from build123d import *

# Parameters (mm, degrees)
EXTRUDE_1_DEPTH     = 6.8
CUT_EXTRUDE_1_DEPTH = 6.9
SKETCH_3_W          = 104
SKETCH_3_H          = 28
EXTRUDE_2_DEPTH     = 32.2
SKETCH_4_W          = 27.8
SKETCH_4_H          = 4.8
CUT_EXTRUDE_2_DEPTH = 6
SKETCH_4_3_W        = 27.8
SKETCH_4_3_H        = 4.8
EXTRUDE_3_DEPTH     = 6
SKETCH_5_W          = 14
SKETCH_5_H          = 14
CUT_EXTRUDE_3_DEPTH = 14
SKETCH_6_R          = 4.2
CUT_EXTRUDE_4_DEPTH = 155.304892988
FILLET_1_R          = 14


with BuildPart() as part:
    # Эскиз1 → Бобышка-Вытянуть1 (new body)
    with BuildSketch(Plane(origin=(0, 0, 0), x_dir=(1, 0, 0), z_dir=(0, 1, 0))):
        with BuildLine():
            ThreePointArc((-28, 0), (0, -28), (28, 0))
            ThreePointArc((28, 0), (11.895099372, 40.186413418), (-28, 57))
            Line((-28, 57), (-140, 57))
            Line((-140, 57), (-140, 29))
            Line((-140, 29), (-36, 29))
            ThreePointArc((-36, 29), (-30.343145751, 26.656854249), (-28, 21))
            Line((-28, 21), (-28, 0))
        make_face()
    extrude(amount=EXTRUDE_1_DEPTH)

    # Эскиз2 → Вырез-Вытянуть1 (cut)
    with BuildSketch(Plane(origin=(0, 6.8, 0), x_dir=(1, 0, 0), z_dir=(0, 1, 0))):
        Polygon((0, 7.15), (-6.192081637, 3.575), (-6.192081637, -3.575), (0, -7.15), (6.192081637, -3.575), (6.192081637, 3.575), align=None)
    extrude(amount=-CUT_EXTRUDE_1_DEPTH, mode=Mode.SUBTRACT)

    # Эскиз3 → Бобышка-Вытянуть2 (add)
    with BuildSketch(Plane(origin=(0, 6.8, 0), x_dir=(1, 0, 0), z_dir=(0, 1, 0))):
        with Locations((-88, 43)):
            Rectangle(SKETCH_3_W, SKETCH_3_H)
    extrude(amount=EXTRUDE_2_DEPTH)

    # Эскиз4 → Вырез-Вытянуть2 (cut)
    with BuildSketch(Plane(origin=(0, 39, 0), x_dir=(1, 0, 0), z_dir=(0, 1, 0))):
        with Locations((-56, 48.6)):
            Rectangle(SKETCH_4_W, SKETCH_4_H)
    extrude(amount=-CUT_EXTRUDE_2_DEPTH, mode=Mode.SUBTRACT)

    # Эскиз4<3> → Бобышка-Вытянуть3 (add)
    with BuildSketch(Plane(origin=(0, 39, 0), x_dir=(1, 0, 0), z_dir=(0, 1, 0))):
        with Locations((-56, 37.4)):
            Rectangle(SKETCH_4_3_W, SKETCH_4_3_H)
    extrude(amount=EXTRUDE_3_DEPTH)

    # Эскиз5 → Вырез-Вытянуть3 (cut)
    with BuildSketch(Plane.XZ):
        with Locations((-126, -43)):
            Rectangle(SKETCH_5_W, SKETCH_5_H)
    extrude(amount=-CUT_EXTRUDE_3_DEPTH, mode=Mode.SUBTRACT)

    # Эскиз6 → Вырез-Вытянуть4 (cut, through all)
    with BuildSketch(Plane.XZ.offset(-14)):
        with Locations(Location((-126, -43, 0), (0, 0, 270))):
            Circle(SKETCH_6_R)
    extrude(amount=-CUT_EXTRUDE_4_DEPTH, mode=Mode.SUBTRACT)

    # Скругление1
    fillet_1_edges = [part.edges().sort_by_distance(p)[0] for p in [
        (-140, 19.5, -29),
        (-140, 19.5, -57),
    ]]
    fillet(fillet_1_edges, radius=FILLET_1_R - 0.0001)  # a hair under: the kernel refuses the full size


solid = part.part
The model under review builds one solid part; all positions refer to its coordinate system, in mm. A direction names the side the tool comes from. Give positions to 0.01 mm unless a question says otherwise; leave off trailing zeros. Order: outer loops, then holes, each group sorted by start corner. A loop starts at its lowest first (then second) coordinate and runs counter-clockwise, first axis right, second up. Notation, with made-up numbers: M -12,-5 L 37,-5 A22 ccw 37,29 Z; hole C -14.5,11.25 d3. An arc over 180 degrees is marked long. Use one line per item in the form item = value. Start each with the question number.
Item 1: For faces 1 (the flat face through (-3.139, 3.448, 5.337)), 2 (the flat face through (-133, 7, -43)), 3 (the flat face through (-56, 45, -37)), 4 (the flat face through (-4, 6.8, -15)), list the 3-axis set-ups (+Z, -Z, +X, -X, +Y, -Y) from which the entire face can be reached by the end or side of a thin tool; tool diameter is ignored.
Item 2: We need section B-B on x = -51.5. Give the boundary of the cut face in (y, z), plus the area to 3 significant figures.
Item 3: Insertion check: pin 1 Ø12 at (x, z) = (-8, -47.5) entering from +Y; pin 2 Ø5.5 at (x, z) = (-59.5, -48.5) entering from +Y; pin 3 Ø3.5 at (y, z) = (2, -1.5) entering from -X. Each pin has a flat end and moves straight along its axis. Give the tip position at first contact, or say it passes through.
Item 4: We need section C-C on y = 5. Give the number of separate pieces and of enclosed holes in the cut face, plus the area to 3 significant figures.
Item 5: To check wall thickness, follow line 1 along Z through (x, y) = (-60, 37); line 2 along X through (y, z) = (20, -43); line 3 along Y through (x, z) = (-2.5, 10). State the ranges of each line that lie inside material, in increasing order. Write a range as from..to.
Item 6: The part is to be moulded in two halves that separate along Z. For faces 5 (the flat face through (-42.1, 42, -37)), 6 (the cylindrical face through (-136, 19.2, -52.8)), 7 (the flat face through (-119, 7, -43)), say which applies: pulls with the +Z half, pulls with the -Z half, needs draft (parallel to the pull), parting line crosses it, or undercut.
Item 7: We need section D-D on z = -32.5. Give the boundary of the cut face in (x, y).
Completed:
q1.face_1 = +Y, -Y
q1.face_2 = -Y
q1.face_3 = +Z, -Z, +X, -X, +Y
q1.face_4 = +Z, -Z, +X, +Y
q2.outline = M 0,-57 L 39,-57 L 39,-51 L 33,-51 L 33,-46.2 L 39,-46.2 L 39,-39.8 L 45,-39.8 L 45,-35 L 39,-35 L 39,-29 L 0,-29 Z
q2.area = 1,090 mm²
q3.pin_1 = 6.8
q3.pin_2 = 39
q3.pin_3 = -28
q4.separate_pieces = 1
q4.enclosed_holes = 2
q4.area = 6,480 mm²
q5.line_1 = -57..-51, -46.2..-29
q5.line_2 = -140..-130.2, -121.8..-36
q5.line_3 = 0..6.8
q6.face_5 = needs draft
q6.face_6 = pulls with the -Z half
q6.face_7 = undercut
q7.outline = M -135.26,0 L 18.21,0 L 18.21,6.8 L -36,6.8 L -36,39 L -135.26,39 Z
